The listing builds one solid part. Answer for the finished solid, in the listing's coordinates (mm). A direction names the side the tool comes from. Coordinates: 2 decimals unless noted, no trailing zeros. Write each loop counter-clockwise with the first axis right and the second up, starting at its lowest first coordinate (ties: lowest second). Pieces come first, ordered by that corner, then holes. Notation, with made-up numbers: M -32.5,42.25 L -18.5,42.25 A15 ccw -18.5,49.25 Z; hole C 66,36 d11. An arc over 180 degrees is marked long. Put each result on its own line as item: value. Start each with the question number.
```python
from build123d import *

# Parameters (mm, degrees)
F0_W      = 50
F0_H      = 90
F1_DEPTH  = 2
F2_R      = 1.5
F3_DEPTH  = 2
F4_W      = 25
F4_H      = 50
F5_DEPTH  = 10
F6_W      = 10
F6_H      = 9
F7_DEPTH  = 15
F8_R      = 1.5
F9_DEPTH  = 3
F10_R     = 1.5
F11_DEPTH = 3
F12_R     = 1
F13_SIZE  = 3


with BuildPart() as f1:
    # F0 (on Top) → F1 (new body)
    with BuildSketch(Plane.XY):
        Rectangle(F0_W, F0_H)
    extrude(amount=F1_DEPTH)

    # F2 (on face) → F3 (cut, through all)
    with BuildSketch(Plane.XY.offset(2)):
        with Locations((-20, 40)):
            Circle(F2_R)
        with Locations((20, 40)):
            Circle(F2_R)
        with Locations((-20, -20.5)):
            Circle(F2_R)
        with Locations((20, -20.5)):
            Circle(F2_R)
    extrude(amount=-F3_DEPTH, mode=Mode.SUBTRACT)

    # F4 (on face) → F5 (join)
    with BuildSketch(Plane.XY.offset(2)):
        Rectangle(F4_W, F4_H)
    extrude(amount=F5_DEPTH)

    # F6 (on face) → F7 (join)
    with BuildSketch(Plane.XY.offset(2)):
        with Locations((0, -40)):
            Rectangle(F6_W, F6_H)
        with Locations((0, 40)):
            Rectangle(F6_W, F6_H)
        with Locations((12, -40)):
            Rectangle(F6_W, F6_H)
        with Locations((-12, -40)):
            Rectangle(F6_W, F6_H)
    extrude(amount=F7_DEPTH)

    # F8 (on face) → F9 (join)
    with BuildSketch(Plane(origin=(0, 44.5, 0), x_dir=(-1, 0, 0), z_dir=(0, 1, 0))):
        with Locations((0, 5.333886)):
            Circle(F8_R)
    extrude(amount=F9_DEPTH)

    # F10 (on face) → F11 (join)
    with BuildSketch(Plane.XZ.offset(44.5)):
        with Locations((0, 7.222579)):
            Circle(F10_R)
        with Locations((-11.5, 7.050698)):
            Circle(F10_R)
        with Locations((11.5, 7.050698)):
            Circle(F10_R)
    extrude(amount=F11_DEPTH)

    # F12
    f12_edges = [f1.edges().sort_by_distance(p)[0] for p in [
        (0, -25, 12),
        (12.5, 0, 12),
        (0, 25, 12),
        (-12.5, 0, 12),
    ]]
    fillet(f12_edges, radius=F12_R)

    # F13
    f13_edges = [f1.edges().sort_by_distance(p)[0] for p in [
        (-12, -44.5, 17),
        (0, -44.5, 17),
        (12, -44.5, 17),
        (0, 44.5, 17),
    ]]
    chamfer(f13_edges, length=F13_SIZE)


solid = f1.part
```
1) A cutting plane is placed at C-C on x = 16. Write down the section's boundary in (y, z), then the cut area to 4 significant figures.
2) A cutting plane is placed at D-D on y = 20.5. Write down the section's boundary in (x, z).
3) Straight lines are drawn through the part: probe 1 along Y at (x, z) = (-4, 8); probe 2 along Y at (x, z) = (1, 8.25); probe 3 along Y at (x, z) = (-12, 10.25). For each, find the intervals that lie inside material, in ascending order.
4) A cutting plane is placed at A-A on y = -20.5. Write down the section's boundary in (x, z).
5) For faces 4 (the face through (5, -40, 9)), 5 (the face through (-12.61, -45.98, 8.06)), 6 (the face through (0, -35.5, 9)), 7 (the face through (0, -45, 1)), determine the directions among +Z, -Z, +X, -X, +Y, -Y from which every point of the face is accessible in a straight line to the end or side of a thin tool.
6) Given pin 1 Ø2.5 at (x, y) = (20, 40) entering from -Z; pin 2 Ø1 at (x, z) = (10, 1) entering from +Y; pin 3 Ø8 at (y, z) = (1, 8) entering from +X; pin 4 Ø2.5 at (y, z) = (-41.5, 9.5) entering from -X, each flat-ended and moving along its own axis, determine where each tip first touches the part or whether it passes through.
7) Determine the mould class of faces 1 (the face through (-25, -1, 1)), 2 (the face through (-21.11, -19.49, 1.01)), 3 (the face through (0, 45, 1)) for opening direction Y: +Y half, -Y half, draft (parallel to the pull), parting line (faces both ways), or undercut.
8) A cutting plane is placed at B-B on x = -20. Write down the section's boundary in (y, z), then the cut area to 3 significant figures.
Answers follow:
1. outline: M -45,0 L 45,0 L 45,2 L -35.5,2 L -35.5,17 L -41.5,17 L -44.5,14 L -44.5,2 L -45,2 Z
1. area: 310.5 mm²
2. outline: M -25,0 L 25,0 L 25,2 L 12.5,2 L 12.5,11 A1 ccw 11.5,12 L -11.5,12 A1 ccw -12.5,11 L -12.5,2 L -25,2 Z
3. probe 1: y = -44.5 to -35.5, -25 to 25, 35.5 to 44.5
3. probe 2: y = -47.5 to -35.5, -25 to 25, 35.5 to 44.5
3. probe 3: y = -44.5 to -35.5, -25 to 25
4. outline: M -25,0 L -21.5,0 L -21.5,2 L -25,2 Z; M -18.5,0 L 18.5,0 L 18.5,2 L 12.5,2 L 12.5,11 A1 ccw 11.5,12 L -11.5,12 A1 ccw -12.5,11 L -12.5,2 L -18.5,2 Z; M 21.5,0 L 25,0 L 25,2 L 21.5,2 Z
5. face 4: +Z, -Y
5. face 5: -Y
5. face 6: +Z, +X, -X
5. face 7: -Z, +X, -X, -Y
6. pin 1: passes through
6. pin 2: stops at y = 45
6. pin 3: stops at x = 12.5
6. pin 4: stops at x = -17
7. face 1: draft
7. face 2: undercut
7. face 3: +Y half
8. outline: M -45,0 L -22,0 L -22,2 L -45,2 Z; M -19,0 L 38.5,0 L 38.5,2 L -19,2 Z; M 41.5,0 L 45,0 L 45,2 L 41.5,2 Z
8. area: 168 mm²
